Design review of the part shown in the three views and the two pictorial views. Dimensions are in mm from the part's minimum x, y and z. A direction names the side the tool comes from. Round coordinates to 2 decimals unless told otherwise and drop trailing zeros. Order: outer loops, then holes, each group sorted by start corner. A loop starts at its lowest first (then second) coordinate and runs counter-clockwise, first axis right, second up.
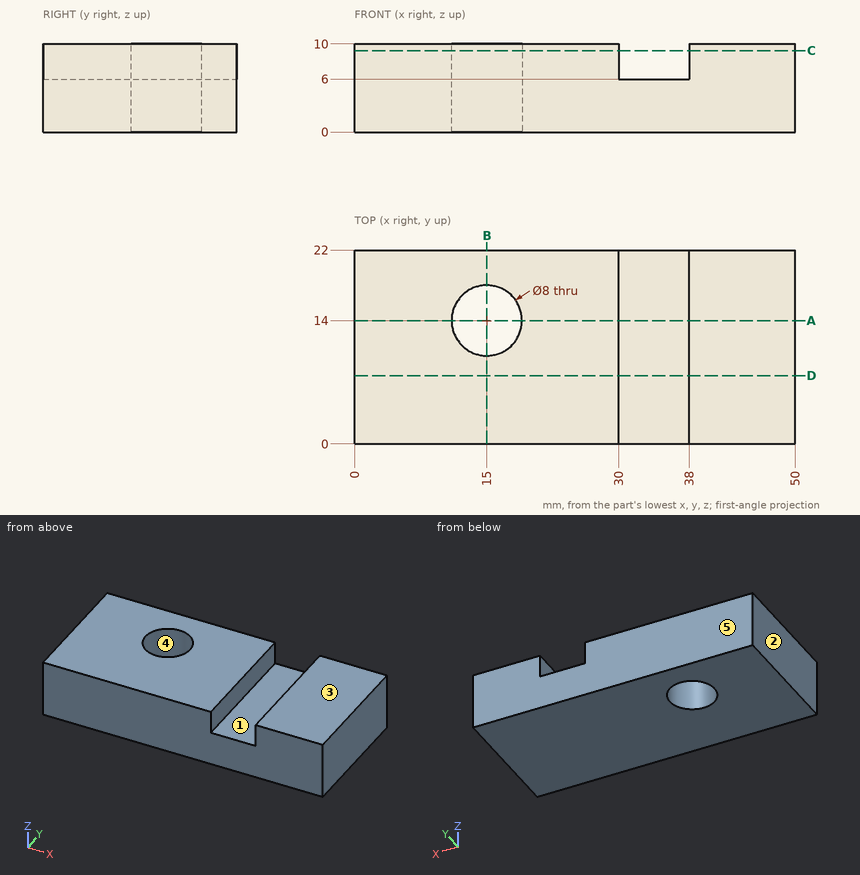
1) The part is to be moulded in two halves that separate along Y. For the marked faces 3, 4 and 5, say which applies: released by +Y, released by -Y, zero draft, split by the parting line, or undercut.
Results:
face 3: zero draft
face 4: undercut
face 5: released by +Y
2) Take a section at C-C on z = 9.25. Give the boundary of the cut face in (x, y).
Results:
outline: (0, 0) - (30, 0) - (30, 22) - (0, 22) - close; (38, 0) - (50, 0) - (50, 22) - (38, 22) - close; hole circle Ø8 at (15, 14)
3) Clearance check with a flat-ended pin moving along its axis: P1, Ø4, axis at x = 32.5, y = 11, coming from the +Z side. State where the tip first meets the part, or that it passes through.
Results:
P1: stops at z = 6
4) Take a section at B-B on x = 15. Give the boundary of the cut face in (y, z).
Results:
outline: (0, 0) - (10, 0) - (10, 10) - (0, 10) - close; (18, 0) - (22, 0) - (22, 10) - (18, 10) - close
5) To check wall thickness, follow line 1 along Y through (x, z) = (15, 2.25); line 2 along Z through (x, y) = (31, 10); line 3 along X through (y, z) = (20, 7.5). State the ranges of each line that lie inside material, in increasing order.
Results:
line 1: y = 0 to 10, 18 to 22
line 2: z = 0 to 6
line 3: x = 0 to 30, 38 to 50
6) For the marked faces 1 and 2, list the 3-axis set-ups (+Z, -Z, +X, -X, +Y, -Y) from which the entire face can be reached by the end or side of a thin tool; tool diameter is ignored.
Results:
face 1: +Z, +Y, -Y
face 2: +Z, -Z, -X, +Y, -Y
7) Take a section at D-D on y = 7.75. Give the boundary of the cut face in (x, z), plus the area to 3 significant figures.
Results:
outline: (0, 0) - (50, 0) - (50, 10) - (38, 10) - (38, 6) - (30, 6) - (30, 10) - (0, 10) - close
area: 468 mm2
8) Take a section at A-A on y = 14. Give the boundary of the cut face in (x, z), plus the area to 3 significant figures.
Results:
outline: (0, 0) - (11, 0) - (11, 10) - (0, 10) - close; (19, 0) - (50, 0) - (50, 10) - (38, 10) - (38, 6) - (30, 6) - (30, 10) - (19, 10) - close
area: 388 mm2
